Can you work these out from the model? Positions are in its coordinate system, mm. Round coordinates to 2 decimals unless told otherwise and drop trailing zeros. Order: outer loops, then holes, each group sorted by start corner. A loop starts at its lowest first (then second) coordinate and runs counter-clockwise, first axis right, second up. Notation, with made-up numbers: (64.5, 50) - (102.5, 50) arc R6 cw to (102.5, 61) - close; hole circle Ø4 at (51, -33). An arc over 180 degrees is marked (long way). Write item = value, one per line.
from build123d import *

# Parameters (mm, degrees)
F0_R     = 1.5
F1_DEPTH = 3


with BuildPart() as f1:
    # F0 (on Top) → F1 (new body)
    with BuildSketch(Plane.XY):
        with BuildLine():
            Line((-15, -6), (-15, 6))
            ThreePointArc((-15, 6), (-21, 0), (-15, -6))
        make_face()
        with Locations((-17.9419908673, 0)):
            Circle(F0_R, mode=Mode.SUBTRACT)
        Polygon((15, 6), (-15, 6), (-15, -6), (15, -6), (15, 1.75009996), (13.512594962, 1.75009996), (13.512594962, -2.7636945222), (12.350259896, -2.7636945222), (12.350259896, 1.75009996), (10.8616553379, 1.75009996), (10.8616553379, 2.7169132347), (15, 2.7169132347), align=None)
        with BuildLine():
            Line((-14.3102758896, -2.7636945222), (-14.3102758896, 2.7169132347))
            Line((-14.3102758896, 2.7169132347), (-12.6045581767, 2.7169132347))
            add(Edge.make_bspline(
                [(-12.6045581767, 2.7169132347), (-11.4386245502, 2.7169132347), (-10.9120351859, 2.3852459016)],
                knots=[0, 0, 0, 1, 1, 1], degree=2))
            add(Edge.make_bspline(
                [(-10.9120351859, 2.3852459016), (-10.3854458217, 2.0535785686), (-10.3854458217, 1.3302678928)],
                knots=[0, 0, 0, 1, 1, 1], degree=2))
            add(Edge.make_bspline(
                [(-10.3854458217, 1.3302678928), (-10.3854458217, 0.8384646142), (-10.6157536985, 0.5235905638)],
                knots=[0, 0, 0, 1, 1, 1], degree=2))
            add(Edge.make_bspline(
                [(-10.6157536985, 0.5235905638), (-10.8460615754, 0.2087165134), (-11.2287085166, 0.1451419432)],
                knots=[0, 0, 0, 1, 1, 1], degree=2))
            Line((-11.2287085166, 0.1451419432), (-11.2287085166, 0.1079568173))
            add(Edge.make_bspline(
                [(-11.2287085166, 0.1079568173), (-10.7081167533, -0.0083966413), (-10.4772091164, -0.3268692523)],
                knots=[0, 0, 0, 1, 1, 1], degree=2))
            add(Edge.make_bspline(
                [(-10.4772091164, -0.3268692523), (-10.2463014794, -0.6453418633), (-10.2463014794, -1.1743302679)],
                knots=[0, 0, 0, 1, 1, 1], degree=2))
            add(Edge.make_bspline(
                [(-10.2463014794, -1.1743302679), (-10.2463014794, -1.9240303878), (-10.7884846062, -2.343862455)],
                knots=[0, 0, 0, 1, 1, 1], degree=2))
            add(Edge.make_bspline(
                [(-10.7884846062, -2.343862455), (-11.3306677329, -2.7636945222), (-12.2602958816, -2.7636945222)],
                knots=[0, 0, 0, 1, 1, 1], degree=2))
            Line((-12.2602958816, -2.7636945222), (-14.3102758896, -2.7636945222))
        make_face(mode=Mode.SUBTRACT)
        with BuildLine():
            add(Edge.make_bspline(
                [(-4.8472610956, 2.0757696921), (-4.1779288285, 1.3482606957), (-4.1779288285, -0.0155937625)],
                knots=[0, 0, 0, 1, 1, 1], degree=2))
            add(Edge.make_bspline(
                [(-4.1779288285, -0.0155937625), (-4.1779288285, -1.3770491803), (-4.8526589364, -2.1081567373)],
                knots=[0, 0, 0, 1, 1, 1], degree=2))
            add(Edge.make_bspline(
                [(-4.8526589364, -2.1081567373), (-5.5273890444, -2.8392642943), (-6.7868852459, -2.8392642943)],
                knots=[0, 0, 0, 1, 1, 1], degree=2))
            add(Edge.make_bspline(
                [(-6.7868852459, -2.8392642943), (-8.0463814474, -2.8392642943), (-8.7211115554, -2.1081567373)],
                knots=[0, 0, 0, 1, 1, 1], degree=2))
            add(Edge.make_bspline(
                [(-8.7211115554, -2.1081567373), (-9.3958416633, -1.3770491803), (-9.3958416633, -0.0083966413)],
                knots=[0, 0, 0, 1, 1, 1], degree=2))
            add(Edge.make_bspline(
                [(-9.3958416633, -0.0083966413), (-9.3958416633, 1.3602558976), (-8.7193122751, 2.0817672931)],
                knots=[0, 0, 0, 1, 1, 1], degree=2))
            add(Edge.make_bspline(
                [(-8.7193122751, 2.0817672931), (-8.0427828868, 2.8032786885), (-6.7796881248, 2.8032786885)],
                knots=[0, 0, 0, 1, 1, 1], degree=2))
            add(Edge.make_bspline(
                [(-6.7796881248, 2.8032786885), (-5.5165933627, 2.8032786885), (-4.8472610956, 2.0757696921)],
                knots=[0, 0, 0, 1, 1, 1], degree=2))
        make_face(mode=Mode.SUBTRACT)
        with BuildLine():
            Line((0.2602958816, 2.7169132347), (1.419032387, 2.7169132347))
            Line((1.419032387, 2.7169132347), (1.419032387, -0.8288684526))
            add(Edge.make_bspline(
                [(1.419032387, -0.8288684526), (1.419032387, -1.4370251899), (1.1473410636, -1.894042383)],
                knots=[0, 0, 0, 1, 1, 1], degree=2))
            add(Edge.make_bspline(
                [(1.1473410636, -1.894042383), (0.8756497401, -2.3510595762), (0.3616553379, -2.5951619352)],
                knots=[0, 0, 0, 1, 1, 1], degree=2))
            add(Edge.make_bspline(
                [(0.3616553379, -2.5951619352), (-0.1523390644, -2.8392642943), (-0.8528588565, -2.8392642943)],
                knots=[0, 0, 0, 1, 1, 1], degree=2))
            add(Edge.make_bspline(
                [(-0.8528588565, -2.8392642943), (-1.9096361455, -2.8392642943), (-2.4944022391, -2.2970811675)],
                knots=[0, 0, 0, 1, 1, 1], degree=2))
            add(Edge.make_bspline(
                [(-2.4944022391, -2.2970811675), (-3.0791683327, -1.7548980408), (-3.0791683327, -0.8144742103)],
                knots=[0, 0, 0, 1, 1, 1], degree=2))
            Line((-3.0791683327, -0.8144742103), (-3.0791683327, 2.7169132347))
            Line((-3.0791683327, 2.7169132347), (-1.9216313475, 2.7169132347))
            Line((-1.9216313475, 2.7169132347), (-1.9216313475, -0.6381447421))
            add(Edge.make_bspline(
                [(-1.9216313475, -0.6381447421), (-1.9216313475, -1.2714914034), (-1.6667333067, -1.5677728908)],
                knots=[0, 0, 0, 1, 1, 1], degree=2))
            add(Edge.make_bspline(
                [(-1.6667333067, -1.5677728908), (-1.4118352659, -1.8640543782), (-0.8228708517, -1.8640543782)],
                knots=[0, 0, 0, 1, 1, 1], degree=2))
            add(Edge.make_bspline(
                [(-0.8228708517, -1.8640543782), (-0.2530987605, -1.8640543782), (0.0035985606, -1.5659736106)],
                knots=[0, 0, 0, 1, 1, 1], degree=2))
            add(Edge.make_bspline(
                [(0.0035985606, -1.5659736106), (0.2602958816, -1.2678928429), (0.2602958816, -0.630947621)],
                knots=[0, 0, 0, 1, 1, 1], degree=2))
            Line((0.2602958816, -0.630947621), (0.2602958816, 2.7169132347))
        make_face(mode=Mode.SUBTRACT)
        Polygon((6.1463414634, -2.7636945222), (2.7612954818, -2.7636945222), (2.7612954818, 2.7169132347), (3.9236305478, 2.7169132347), (3.9236305478, -1.8040783687), (6.1463414634, -1.8040783687), align=None, mode=Mode.SUBTRACT)
        Polygon((10.2546981208, -1.8040783687), (10.2546981208, -2.7636945222), (7.0987604958, -2.7636945222), (7.0987604958, 2.7169132347), (10.2546981208, 2.7169132347), (10.2546981208, 1.7644942023), (8.2610955618, 1.7644942023), (8.2610955618, 0.5613754498), (10.1167532987, 0.5613754498), (10.1167532987, -0.3910435826), (8.2610955618, -0.3910435826), (8.2610955618, -1.8040783687), align=None, mode=Mode.SUBTRACT)
        with BuildLine():
            ThreePointArc((15, -6), (21, 0), (15, 6))
            Line((15, 6), (15, 2.7169132347))
            Line((15, 2.7169132347), (15, 1.75009996))
            Line((15, 1.75009996), (15, -6))
        make_face()
    extrude(amount=F1_DEPTH)


solid = f1.part
(1) Thinking about a two-plate mould opening in X: for faces 1 (the face through (9, -0.391, 1)), 2 (the face through (-21, 0, 1)), which applies, +X half, -X half, draft (parallel to the pull), parting line (faces both ways), or undercut?
Computed:
face_1 = undercut
face_2 = -X half
(2) If we section it at A-A (z = 1.7): State how many separate pieces and enclosed holes the cut face has, plus the area to 3 significant figures.
Computed:
separate_pieces = 1
enclosed_holes = 7
area = 378 mm^2
(3) If we section it at C-C (y = 3.25): Write out the boundary of the cut face in (x, z), plus the area to 3 significant figures.
Computed:
outline = (-20.04, 0) - (20.04, 0) - (20.04, 3) - (-20.04, 3) - close
area = 120 mm^2
(4) Will these pins go through, and if not, where does the flat tip stop? P1, Ø0.5, axis at y = 2, z = 1.5, coming from the -X side; P2, Ø1, axis at y = 4.5, z = 1.5, coming from the +X side; P3, Ø0.6, axis at y = 1, z = 2, coming from the -X side.
Computed:
P1 = -20.74
P2 = 19.47
P3 = -20.96
(5) If I drill on line 1 (Y direction, x = 14, z = 1.5); line 2 (Y direction, x = -10.5, z = 0.8); line 3 (Y direction, x = 6, z = 2.7), over which ranges is the centre line in solid material (lowest first)? Write a range as from..to.
Computed:
line_1 = -6..1.75, 2.72..6
line_2 = -6..-2.05, -0.3..0.72, 1.92..6
line_3 = -6..-2.76, -1.8..6
(6) If we section it at B-B (y = -4): Write out the boundary of the cut face in (x, z), plus the area to 3 significant figures.
Computed:
outline = (-19.47, 0) - (19.47, 0) - (19.47, 3) - (-19.47, 3) - close
area = 117 mm^2
